from build123d import *

# Parameters (mm, degrees)
F0_W      = 40
F0_H      = 40
F1_DEPTH  = 1900
F3_DEPTH  = 40.001
F4_W      = 48
F4_H      = 214.6480633261
F5_DEPTH  = 5
F6_W      = 48
F6_H      = 150
F7_DEPTH  = 5
F8_R      = 4.5
F9_DEPTH  = 5
F10_R     = 4.5
F11_DEPTH = 5
F12_R     = 5


with BuildPart() as f1:
    # F0 (on Front) → F1 (new body)
    with BuildSketch(Plane.XZ):
        Rectangle(F0_W, F0_H)
    extrude(amount=F1_DEPTH)

    # F2 (on face) → F3 (cut, through all)
    with BuildSketch(Plane(origin=(-20, 0, 0), x_dir=(0, -1, 0), z_dir=(-1, 0, 0))):
        Polygon((85.7802768204, 20), (0, 20), (0, -20), align=None)
        Polygon((1900, -20), (1900, 20), (1881.3476936738, 20), align=None)
    extrude(amount=-F3_DEPTH, mode=Mode.SUBTRACT)

    # F4 (on face) → F5 (join)
    with BuildSketch(Plane(origin=(0, -7.6604444312, -16.4278760969), x_dir=(1, 0, 0), z_dir=(0, 0.4226182617, 0.906307787))):
        with Locations((0, -58.8716664282)):
            Rectangle(F4_W, F4_H)
    extrude(amount=F5_DEPTH)

    # F6 (on face) → F7 (join)
    with BuildSketch(Plane(origin=(0, -1552.987784771, 724.1700970599), x_dir=(1, 0, 0), z_dir=(0, -0.906307787, 0.4226182617))):
        with Locations((0, -799.0332946688)):
            Rectangle(F6_W, F6_H)
    extrude(amount=F7_DEPTH)

    # F8 (on face) → F9 (cut, through all)
    with BuildSketch(Plane(origin=(0, -1557.5193237062, 726.2831883686), x_dir=(1, 0, 0), z_dir=(0, -0.906307787, 0.4226182617))):
        with Locations((0, -859.0332946688)):
            Circle(F8_R)
        with Locations((0, -739.0332946688)):
            Circle(F8_R)
    extrude(amount=-F9_DEPTH, mode=Mode.SUBTRACT)

    # F10 (on face) → F11 (cut, through all)
    with BuildSketch(Plane(origin=(0, -5.5473531225, -11.8963371617), x_dir=(1, 0, 0), z_dir=(0, 0.4226182617, 0.906307787))):
        with Locations((0, 28.4523652348)):
            Circle(F10_R)
        with BuildLine():
            Line((-4.5, -146.1956980913), (4.5, -146.1956980913))
            ThreePointArc((4.5, -146.1956980913), (0, -141.6956980913), (-4.5, -146.1956980913))
        make_face()
        with BuildLine():
            ThreePointArc((-4.5, -146.1956980913), (0, -150.6956980913), (4.5, -146.1956980913))
            Line((4.5, -146.1956980913), (-4.5, -146.1956980913))
        make_face()
        with BuildLine():
            ThreePointArc((-4.5, -146.1956980913), (0, -141.6956980913), (4.5, -146.1956980913))
            Line((4.5, -146.1956980913), (4.5, -116.1956980913))
            Line((4.5, -116.1956980913), (-4.5, -116.1956980913))
            Line((-4.5, -116.1956980913), (-4.5, -146.1956980913))
        make_face()
        with BuildLine():
            Line((-4.5, -116.1956980913), (4.5, -116.1956980913))
            ThreePointArc((4.5, -116.1956980913), (0, -111.6956980913), (-4.5, -116.1956980913))
        make_face()
    extrude(amount=-F11_DEPTH, mode=Mode.SUBTRACT)

    # F12
    f12_edges = [f1.edges().sort_by_distance(p)[0] for p in [
        (-24, 37.308857, -34.638961),
        (-24, -157.228354, 56.07523),
        (24, 37.308857, -34.638961),
        (24, -157.228354, 56.07523),
        (-24, -1924.635986, -66.916538),
        (24, -1924.635986, -66.916538),
        (24, -1861.243247, 69.02963),
        (-24, -1861.243247, 69.02963),
    ]]
    fillet(f12_edges, radius=F12_R)


solid = f1.part
The model under review builds one solid part; all positions refer to its coordinate system, in mm. Coordinates: 2 decimals unless noted, no trailing zeros. Loops run counter-clockwise (first coordinate to the right, second up) from the corner with the lowest first, then second, coordinate; pieces in that order, holes last. Notation, with made-up numbers: M 37.25,10 L 80.25,10 A24 cw 80.25,32 Z; hole C -24.75,18.5 d8. An arc over 180 degrees is marked long. Put each result on its own line as item: value. Start each with the question number.
Q1. Wall thickness on line 1 (Z direction, x = -1, y = -883.5); line 2 (Y direction, x = -2, z = 48): over which ranges is each line inside the solid? List them lowest first.
Q2. Add section A-A (z = 3.5). Write out the cut boundary in (x, y).
Q3. The part is to be moulded in two halves that separate along Z. For faces 1 (the flat face through (-0.336, -1894.762, 3.065)), 2 (the flat face through (0, -937, -20)), 3 (the flat face through (-24, -1893, 0)), 4 (the flat face through (21, -1890.23, 0.95)), say which applies: +Z half, -Z half, draft (parallel to the pull), parting line (faces both ways), or undercut.
Q4. Clearance check with flat-ended pins moving along their axes: pin 1 (12 mm diameter, centred on y = -1318, z = 8.5, fed in from +X); pin 2 (1.5 mm diameter, centred on x = 18, z = -49.5, fed in from +Y); pin 3 (5 mm diameter, centred on x = 18, y = -331.5, fed in from +Z). State where each tip first meets the part, or that it passes through.
Q5. Add section B-B (y = -508). Write out the cut boundary in (x, z).
Answers:
1. line 1: z = -20 to 20
1. line 2: y = -1873.81 to -1868.29, -145.83 to -143.37
2. outline: M -24,-1894.56 L 24,-1894.56 L 24,-1889.04 L 20,-1889.04 L 20,-50.4 L 24,-50.4 L 24,-38.56 L -24,-38.56 L -24,-50.4 L -20,-50.4 L -20,-1889.04 L -24,-1889.04 Z
3. face 1: +Z half
3. face 2: -Z half
3. face 3: draft
3. face 4: undercut
4. pin 1: stops at x = 20
4. pin 2: stops at y = -1913.41
4. pin 3: stops at z = 20
5. outline: M -20,-20 L 20,-20 L 20,20 L -20,20 Z
